Geometry: final body of the model. Coordinates: model frame, mm. Face numbers are marked on the shaded views. A direction names the side the tool comes from. Give positions to 0.01 mm unless a question says otherwise; leave off trailing zeros. Write each loop counter-clockwise with the first axis right and the second up, starting at its lowest first coordinate (ties: lowest second). Pieces come first, ordered by that corner, then holes. Notation, with made-up numbers: M 44,-28.75 L 68,-28.75 A21 ccw 68,7.25 Z; hole C 82,22 d8. An arc over 180 degrees is marked long. Use one line per item in the form item = value. Start each with the question number.
Item 1: Pull-direction query (X, two-part tool) for the marked faces 4, 5 and 6; classes: released by +X, released by -X, zero draft, split by the parting line, or undercut.
Item 2: Section query C-C on z = 12.5. Return loops of the section in (x, y).
Item 3: Material intervals for line 1 along X through (y, z) = (2, 10.25); line 2 along Y through (x, z) = (-4, 7.75); line 3 along X through (y, z) = (14.5, 22), sorted ascending. Write a range as from..to.
Item 4: Section query D-D on z = 9.75. Return loops of the section in (x, y).
Item 5: Access query for the marked faces 1, 2 and 3. Directions: +Z, -Z, +X, -X, +Y, -Y. A direction counts if a zero-diameter tool reaches every point of the face in a straight line with its end or side. Return the directions, or none.
Item 6: Section query A-A on z = 21.25. Return loops of the section in (x, y).
Item 7: Section query B-B on x = -6.25. Return loops of the section in (y, z).
Item 8: Contact query for flat-ended pins moving along their axis: P1, Ø5, axis at y = 15.5, z = 22.5, coming from the -X side; P2, Ø4, axis at y = 10, z = 5.5, coming from the -X side; P3, Ø4, axis at x = -2.5, z = 8, coming from the +Y side; P4, Ø3, axis at y = 13.88, z = 12.5, coming from the +X side. Output: stop coordinate, or through.
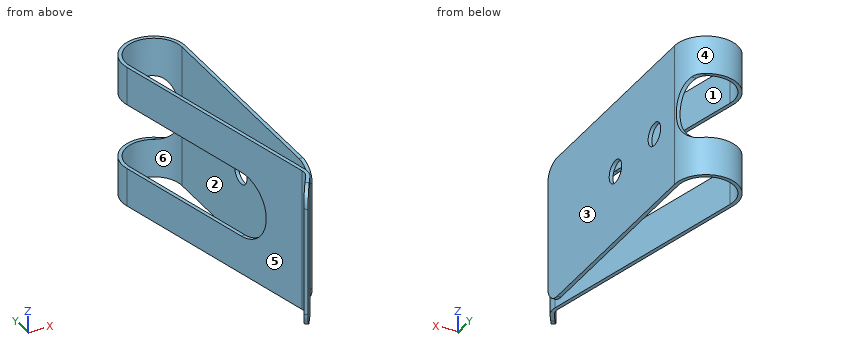
from build123d import *

# Parameters (mm, degrees)
EXTRUDE_THIN1_DEPTH              = 25
CUT_EXTRUDE1_REACH               = 41.464
CUT_EXTRUDE1_OFFSET_FROM_SURFACE = 2
CUT_EXTRUDE2_DEPTH               = 39.114790536728684
CUT_EXTRUDE2_DEPTH_BACK          = 39.114790536728684
FILLET1_R                        = 2
FILLET2_R                        = 3
SKETCH4_R                        = 1.9999999999999996
CUT_EXTRUDE3_DEPTH               = 39.11479062976518


with BuildPart() as part:
    # Sketch1 → Extrude-Thin1 (new body)
    with BuildSketch(Plane.XY):
        with BuildLine():
            Line((-3.622105329640586, -26.801338649985606), (-1.0941188006005313, -22.79472249406353))
            ThreePointArc((-1.0941188006005313, -22.79472249406353), (-0.66792233314523, -21.684442737284584), (-0.6990538082442912, -20.49557966760723))
            Line((-0.6990538082442912, -20.49557966760723), (-9.68971050504969, 19.237405741595826))
            ThreePointArc((-9.68971050504969, 19.237405741595826), (-5.449997394886004, 25.195000000000007), (0, 20.320000000000004))
            Line((0, 20.320000000000004), (0, -20.320000000000004))
            Line((0, -20.320000000000004), (0.65, -20.320000000000004))
            Line((0.65, -20.320000000000004), (0.65, 20.320000000000004))
            ThreePointArc((0.6499999999999986, 20.320000000000004), (-5.52217034544628, 25.840980700336655), (-10.323683013380226, 19.093952408831854))
            Line((-10.323683013380226, 19.093952408831854), (-1.3330263165748255, -20.639033000371203))
            ThreePointArc((-1.3330263165748275, -20.639033000371192), (-1.3085337715329808, -21.57436555978272), (-1.6438418847081215, -22.4478730587184))
            Line((-1.6438418847081135, -22.447873058718383), (-4.171828413748168, -26.454489214640457))
            Line((-4.171828413748168, -26.454489214640457), (-3.622105329640586, -26.801338649985606))
        make_face()
    extrude(amount=EXTRUDE_THIN1_DEPTH)

    # Cut-Extrude1: up to this face of the body (flat: up to its plane, moved by the offset)
    cut_extrude1_end = Plane(part.part.faces().sort_by_distance((0, 0, 12.5))[0]).offset(CUT_EXTRUDE1_OFFSET_FROM_SURFACE)
    # Sketch2 → Cut-Extrude1 (cut, up to the picked face)
    with BuildSketch(Plane(origin=(-5.7107644938092665, -1.2922140763239114, 0), x_dir=(0, 0, 1), z_dir=(-0.9753423205085142, -0.22069743502149478, 0)), mode=Mode.PRIVATE) as cut_extrude1_sk1:
        with BuildLine():
            Line((18.249999999999996, 28.456882519592593), (18.25, -5.793117480407402))
            ThreePointArc((18.25, -5.793117480407402), (12.499999999999998, -11.5431174804074), (6.750000000000001, -5.793117480407404))
            Line((6.750000000000001, -5.793117480407404), (6.749999999999996, 28.456882519592593))
            ThreePointArc((6.749999999999996, 28.456882519592593), (12.499999999999995, 34.2068825195926), (18.249999999999996, 28.456882519592593))
        make_face()
    cut_extrude1_tool1 = split(extrude(cut_extrude1_sk1.sketch, amount=-CUT_EXTRUDE1_REACH, mode=Mode.PRIVATE), bisect_by=cut_extrude1_end, keep=Keep.BOTH, mode=Mode.PRIVATE)
    add(cut_extrude1_tool1.solids().sort_by(Axis((-8.211682, 9.760251, 12.5), (0.9753423205085142, 0.22069743502149478, 0)))[0], mode=Mode.SUBTRACT)

    # Sketch3 → Cut-Extrude2 (cut, two sides: drawn at the far end of the back side and taken through both)
    with BuildSketch(Plane.ZY.offset(-CUT_EXTRUDE2_DEPTH_BACK)):
        with BuildLine():
            Line((18.249999999999993, 24.27238272866149), (18.249999999999996, 25.05505662424576))
            Line((18.249999999999996, 25.05505662424576), (6.749999999999996, 25.05505662424576))
            Line((6.749999999999996, 25.05505662424576), (6.749999999999999, 24.27238272866149))
            ThreePointArc((6.749999999999999, 24.27238272866149), (12.499999999999995, 20.875332308455405), (18.249999999999993, 24.27238272866149))
        make_face()
    extrude(amount=CUT_EXTRUDE2_DEPTH + CUT_EXTRUDE2_DEPTH_BACK, mode=Mode.SUBTRACT)

    # Fillet1
    # the kernel refuses this fillet: 2 mm, written as the material it adds along each edge
    with BuildSketch(Plane(origin=(0.6919383663248766, 24.272382728661498, 18.25), x_dir=(0, -0.8498127825413853, -0.5270846560366448), z_dir=(-1, 0, 0))) as fillet1_piece_1_section:
        with BuildLine():
            CenterArc((0.5741727604103483, -1.997336805169661), FILLET1_R, 87.04285714004924, 34.765830441625596)
            Line((-0.47999655166291116, -0.29771124008687166), (0, 0))
            ThreePointArc((0, 0), (0.3386753487804471, 0.00874177622603999), (0.6773506975608955, 0))
        make_face()
    fillet1_piece_1 = extrude(amount=4.385315110227097, mode=Mode.PRIVATE)
    fillet1_piece_1 = fillet1_piece_1 & Plane(origin=(-4.905332308455408, 20.320000000000007, 18.185221139731127), x_dir=(1, -6.4e-16, 0), z_dir=(0, 0, -1)) * Cylinder(5.555332308455408, 12, mode=Mode.PRIVATE)
    fillet1_piece_1 = fillet1_piece_1 - Plane(origin=(-4.90533230845541, 20.320000000000007, 18.185221139731127), x_dir=(-0.9753423205085139, -0.220697435021496, 0), z_dir=(0, 0, -1)) * Cylinder(4.9053323084554075, 12, mode=Mode.PRIVATE)
    add(fillet1_piece_1)
    with BuildSketch(Plane(origin=(-3.6933767439022205, 24.272382728661498, 6.7499999999999964), x_dir=(0, 1, 0), z_dir=(1, 0, 0))) as fillet1_piece_2_section:
        with BuildLine():
            CenterArc((0.5648262317583601, 2), FILLET1_R, 235.23416955837342, 34.765830441626576)
            ThreePointArc((-0.5756212810506085, 0.35702115944001456), (-0.2924182966405411, 0.17108170654102572), (0, 0))
            Line((0, 0), (0.5648262317583601, 0))
        make_face()
    fillet1_piece_2 = extrude(amount=4.385315110227104, mode=Mode.PRIVATE)
    fillet1_piece_2 = fillet1_piece_2 - Plane(origin=(-4.90533230845541, 20.320000000000007, 6.814778786528934), x_dir=(-0.9753423205085139, -0.220697435021496, 0), z_dir=(0, 0, -1)) * Cylinder(4.9053323084554075, 12, mode=Mode.PRIVATE)
    fillet1_piece_2 = fillet1_piece_2 & Plane(origin=(-4.905332308455408, 20.320000000000007, 6.814778786528934), x_dir=(1, -6.4e-16, 0), z_dir=(0, 0, -1)) * Cylinder(5.555332308455408, 12, mode=Mode.PRIVATE)
    add(fillet1_piece_2)

    # Fillet2
    fillet2_edges = [part.edges().sort_by_distance(p)[0] for p in [
        (0.325, -20.320000000000004, 0),
        (-3.896966871694377, -26.62791393231303, 0),
        (0.325, -20.320000000000004, 25),
        (-3.896966871694377, -26.62791393231303, 25),
    ]]
    fillet(fillet2_edges, radius=FILLET2_R)

    # Sketch4 → Cut-Extrude3 (cut, through all)
    with BuildSketch(Plane.ZY):
        with Locations(Location((12.5, 13.875332308455407, 0), (0, 0, 270))):
            Circle(SKETCH4_R)
        with Locations(Location((12.5, 1.375332308455407, 0), (0, 0, 270))):
            Circle(SKETCH4_R)
    extrude(amount=-CUT_EXTRUDE3_DEPTH, mode=Mode.SUBTRACT)


solid = part.part
Answer sheet:
q1.face_4 = split by the parting line
q1.face_5 = released by -X
q1.face_6 = undercut
q2.outline = M -4.17,-26.45 L -3.62,-26.8 L -1.09,-22.79 A3.05 ccw -0.7,-20.5 L -2.53,-12.41 L -3.16,-12.55 L -1.33,-20.64 A2.4 cw -1.64,-22.45 Z; M -0.03,20.88 A4.91 cw 0,20.32 L 0,15.88 L 0.65,15.88 L 0.65,20.32 A5.56 ccw 0.62,20.88 Z; M 0,-20.32 L 0.65,-20.32 L 0.65,-0.62 L 0,-0.62 Z; M 0,3.38 L 0.65,3.38 L 0.65,11.88 L 0,11.88 Z
q3.line_1 = 0..0.65
q3.line_2 = -26.56..-26.18
q3.line_3 = -9.28..-8.62, 0..0.65
q4.outline = M -4.17,-26.45 L -3.62,-26.8 L -1.09,-22.79 A3.05 ccw -0.7,-20.5 L -2.68,-11.72 L -3.32,-11.87 L -1.33,-20.64 A2.4 cw -1.64,-22.45 Z; M -0.14,21.48 A4.91 cw 0,20.32 L 0,-20.32 L 0.65,-20.32 L 0.65,20.32 A5.56 ccw 0.53,21.48 Z
q5.face_1 = +Z, -Z
q5.face_2 = +Z, -Z, -Y
q5.face_3 = +Z, -Z, +X, +Y, -Y
q6.outline = M -10.32,19.09 L -1.33,-20.64 A2.4 cw -1.64,-22.45 L -4.17,-26.45 L -3.62,-26.8 L -1.09,-22.79 A3.05 ccw -0.7,-20.5 L -9.69,19.24 A4.91 cw long 0,20.32 L 0,-20.32 L 0.65,-20.32 L 0.65,20.32 A5.56 ccw long Z
q7.outline = M 1.09,0 L 4.04,0 L 4.04,6.75 L 1.09,6.75 Z; M 1.09,18.25 L 4.04,18.25 L 4.04,25 L 1.09,25 Z; M 25.04,0 L 25.71,0 L 25.71,6.75 L 25.04,6.75 Z; M 25.04,18.25 L 25.71,18.25 L 25.71,25 L 25.04,25 Z
q8.P1 = -10.08
q8.P2 = -8.72
q8.P3 = 25.81
q8.P4 = through
